```python
from build123d import *

# Parameters (mm, degrees)
SKETCH1_W           = 25
SKETCH1_H           = 25
BOSS_EXTRUDE1_DEPTH = 50
CUT_EXTRUDE2_REACH  = 111.973
CUT_EXTRUDE3_REACH  = 111.973
SKETCH3_W           = 19
SKETCH3_H           = 12
SKETCH1_3_W         = 25
SKETCH1_3_H         = 25
BOSS_EXTRUDE2_DEPTH = 31
CUT_EXTRUDE4_REACH  = 102.305
SKETCH4_W           = 25
SKETCH4_H           = 0.253333333


with BuildPart() as part:
    # Sketch1 → Boss-Extrude1 (new body)
    with BuildSketch(Plane(origin=(0, 0, 0), x_dir=(1, 0, 0), z_dir=(0, 1, 0))):
        Polygon((0, 0), (25, 0), (25, 15), (50, 15), (50, 0), (75, 0), (75, 63), (0, 63), align=None)
        with Locations((24.5, 31.5)):
            Rectangle(SKETCH1_W, SKETCH1_H, mode=Mode.SUBTRACT)
    extrude(amount=BOSS_EXTRUDE1_DEPTH)

    # Sketch2 → Cut-Extrude2 (cut, up to next)
    with BuildSketch(Plane(origin=(0, 0, -63), x_dir=(-1, 0, 0), z_dir=(0, 0, -1)), mode=Mode.PRIVATE) as cut_extrude2_sk1:
        Polygon((0, 12), (-75, 50), (0, 50), align=None)
    cut_extrude2_tool1 = extrude(cut_extrude2_sk1.sketch, amount=-CUT_EXTRUDE2_REACH, mode=Mode.PRIVATE) & part.part
    add(cut_extrude2_tool1.solids().sort_by_distance((25, 37.333333, -63))[0], mode=Mode.SUBTRACT)

    # Sketch3 → Cut-Extrude3 (cut, up to next)
    with BuildSketch(Plane(origin=(75, 0, 0), x_dir=(0, 0, -1), z_dir=(1, 0, 0)), mode=Mode.PRIVATE) as cut_extrude3_sk1:
        with Locations((31.5, 44)):
            Rectangle(SKETCH3_W, SKETCH3_H)
    cut_extrude3_tool1 = extrude(cut_extrude3_sk1.sketch, amount=-CUT_EXTRUDE3_REACH, mode=Mode.PRIVATE) & part.part
    add(cut_extrude3_tool1.solids().sort_by_distance((75, 44, -31.5))[0], mode=Mode.SUBTRACT)

    # Sketch1<3> → Boss-Extrude2 (add)
    with BuildSketch(Plane(origin=(0, 0, 0), x_dir=(1, 0, 0), z_dir=(0, 1, 0))):
        with Locations((24.5, 31.5)):
            Rectangle(SKETCH1_3_W, SKETCH1_3_H)
    extrude(amount=BOSS_EXTRUDE2_DEPTH)

    # Sketch4 → Cut-Extrude4 (cut, up to next)
    with BuildSketch(Plane.XY.offset(-19), mode=Mode.PRIVATE) as cut_extrude4_sk1:
        with Locations((24.5, 30.873333334)):
            Rectangle(SKETCH4_W, SKETCH4_H)
    cut_extrude4_tool1 = extrude(cut_extrude4_sk1.sketch, amount=-CUT_EXTRUDE4_REACH, mode=Mode.PRIVATE) & part.part
    add(cut_extrude4_tool1.solids().sort_by_distance((24.5, 30.873333, -19))[0], mode=Mode.SUBTRACT)


solid = part.part
```
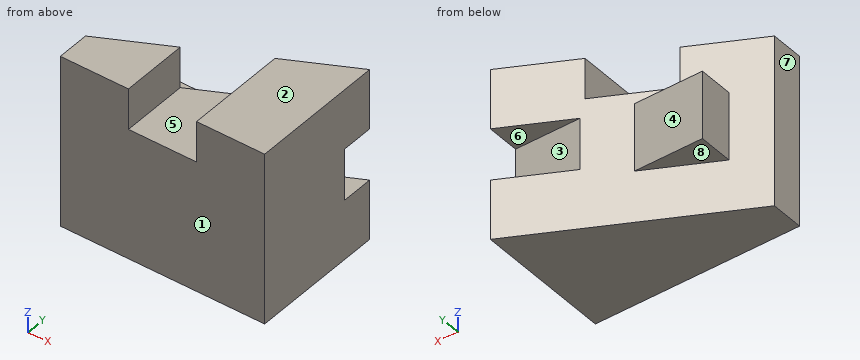
Geometry: final body of the model. Coordinates: model frame, mm. Face numbers are marked on the shaded views. A direction names the side the tool comes from. Coordinates: 2 decimals unless noted, no trailing zeros. Order: outer loops, then holes, each group sorted by start corner. A loop starts at its lowest first (then second) coordinate and runs counter-clockwise, first axis right, second up. Notation, with made-up numbers: (-3, 84.5) -> (47, 84.5) arc R9 ccw to (47, 95.5) -> close; hole circle Ø8 at (18.25, -2.5). An arc over 180 degrees is marked (long way). Answer in a Markdown table with one row per item.
Item 1: Access query for the marked faces 4, 5, 6, 7 and 8. Directions: +Z, -Z, +X, -X, +Y, -Y. A direction counts if a zero-diameter tool reaches every point of the face in a straight line with its end or side. Return the directions, or none.
Return value:
| item | result |
|---|---|
| face 4 | +Z, -Z, -X, +Y |
| face 5 | +Z, +Y, -Y |
| face 6 | +X, -X, +Y |
| face 7 | +Z, -Z, -X, +Y, -Y |
| face 8 | -Z, -X, +Y |
Item 2: Ray query, L1, parallel to X at y = 9, z = -13; L2, parallel to Z at x = 40, y = 20; L3, parallel to Y at x = 27.5, z = -24. Return the intervals inside material, ascending.
Return value:
| item | result |
|---|---|
| L1 | x = 0 to 25, 50 to 75 |
| L2 | z = -63 to -15 |
| L3 | y = 0 to 30.75 |
Item 3: Contact query for flat-ended pins moving along their axis: P1, Ø12.5, axis at x = 29, z = -33.5, coming from the +Y side; P2, Ø4.5, axis at y = 20, z = -7, coming from the -X side; P3, Ø6, axis at y = 45, z = -10.5, coming from the -X side. Output: stop coordinate, or through.
Return value:
| item | result |
|---|---|
| P1 | stops at y = 30.75 |
| P2 | stops at x = 11.35 |
| P3 | stops at x = 59.21 |
Item 4: Section B-B on x = 30. Output: boundary loops of the cut face in (y, z).
Return value:
| item | result |
|---|---|
| outline | (0, -63) -> (27.2, -63) -> (27.2, -44) -> (30.75, -44) -> (30.75, -19) -> (27.2, -19) -> (27.2, -15) -> (0, -15) -> close |
Item 5: Section A-A on z = -5. Output: boundary loops of the cut face in (x, y), plus the area to 3 significant figures.
Return value:
| item | result |
|---|---|
| outline | (0, 0) -> (25, 0) -> (25, 24.67) -> (0, 12) -> close; (50, 0) -> (75, 0) -> (75, 50) -> (50, 37.33) -> close |
| area | 1,550 mm² |
Item 6: Section C-C on y = 10. Output: boundary loops of the cut face in (x, z), plus the area to 3 significant figures.
Return value:
| item | result |
|---|---|
| outline | (0, -63) -> (75, -63) -> (75, 0) -> (50, 0) -> (50, -15) -> (25, -15) -> (25, 0) -> (0, 0) -> close |
| area | 4,350 mm² |
Item 7: Draft query along Z for the marked faces 1, 2 and 3. Return one class per face: released by +Z, released by -Z, zero draft, split by the parting line, or undercut.
Return value:
| item | result |
|---|---|
| face 1 | zero draft |
| face 2 | released by +Z |
| face 3 | undercut |
Item 8: Section D-D on y = 44. Output: boundary loops of the cut face in (x, z), plus the area to 3 significant figures.
Return value:
| item | result |
|---|---|
| outline | (63.16, -63) -> (75, -63) -> (75, -41) -> (63.16, -41) -> close; (63.16, -22) -> (75, -22) -> (75, 0) -> (63.16, 0) -> close |
| area | 521 mm² |
